Verification items for the finished model (mm, model axes). A direction names the side the tool comes from. Coordinates: 2 decimals unless noted, no trailing zeros. Loops run counter-clockwise (first coordinate to the right, second up) from the corner with the lowest first, then second, coordinate; pieces in that order, holes last. Notation, with made-up numbers: (63, 55.5) -> (105, 55.5) arc R19 ccw to (105, 82.5) -> close; hole circle Ø7 at (26, -5.75). An arc over 180 degrees is marked (long way). Answer as a JSON object with one key per item and string values. Group by question number.
Q1. Cross-section at C-C on y = 3053.5. Record the boundary of the cut face in (x, z).
Q2. Cross-section at B-B on x = 1900. Record the boundary of the cut face in (y, z).
Q3. Scan lines: L1, parallel to X at y = 3044.5, z = 2.9; L2, parallel to X at y = 3161, z = 3.2; L3, parallel to X at y = 2953, z = 4.55. Record each from-to range of solid material in increasing order.
Q4. Gauge pin test, flat ends, axial feed: pin 1 Ø3.5 at (x, y) = (1920.9, 2839.09) entering from +Z; pin 2 Ø2.5 at (x, z) = (1510, 3) entering from +Y; pin 3 Ø2.5 at (x, z) = (1641, 1.5) entering from -Y; pin 4 Ø1.5 at (x, z) = (1655, 3.5) entering from -Y. Record the tip position at first contact, or that the pin passes through.
Q5. Set-up check for faces 1 (the cylindrical face through (1470.405, 3112.471, 2.465)), 2 (the flat face through (1816.93, 3217.31, 2.46)): record each of +Z, -Z, +X, -X, +Y, -Y from which the full face is reachable in a straight line by a thin tool's end or side.
Q6. Cross-section at A-A on y = 3282. Give the number of separate pieces and of enclosed holes in the cut face, and give its area (3 significant figures).
```python
from build123d import *

# Parameters (mm, degrees)
MODEL_R         = 3
MODEL_R_2       = 2.999999999
EXTRUDE_1_DEPTH = 5


with BuildPart() as part:
    # Model → 凸台-拉伸1 (new body)
    with BuildSketch(Plane.XY):
        with BuildLine():
            Line((1801.04667122, 3384.62585133), (1652.053473941, 3384.62585133))
            ThreePointArc((1652.053473941, 3384.62585133), (1476.211681089, 3361.037418459), (1452.966845602, 3185.14987512))
            ThreePointArc((1452.966845602, 3185.14987512), (1470.408197338, 3111.400724011), (1452.966841198, 3037.651573943))
            ThreePointArc((1452.966841198, 3037.651573943), (1476.211684212, 2861.76403514), (1652.053473941, 2838.175605395))
            Line((1652.053473941, 2838.175605395), (1801.04667122, 2838.175605395))
            ThreePointArc((1801.04667122, 2838.175605395), (1976.888464071, 2861.764038266), (2000.13329956, 3037.651581604))
            ThreePointArc((2000.13329956, 3037.651581604), (1980.450087896, 3111.400728363), (2000.13329956, 3185.149875122))
            ThreePointArc((2000.13329956, 3185.149875122), (1976.888464071, 3361.037418459), (1801.04667122, 3384.62585133))
        make_face()
        with Locations((1463.462548046, 3185.149875121)):
            Circle(MODEL_R, mode=Mode.SUBTRACT)
        with Locations((1447.208426339, 3293.322313167)):
            Circle(MODEL_R, mode=Mode.SUBTRACT)
        with Locations((1525.324154834, 3383.712293191)):
            Circle(MODEL_R, mode=Mode.SUBTRACT)
        with Locations((1463.462548046, 3037.651582732)):
            Circle(MODEL_R, mode=Mode.SUBTRACT)
        with Locations((1447.208426339, 2929.479144686)):
            Circle(MODEL_R, mode=Mode.SUBTRACT)
        with Locations((1525.324154834, 2839.089164661)):
            Circle(MODEL_R, mode=Mode.SUBTRACT)
        with Locations((1991.691967871, 3185.149875121)):
            Circle(MODEL_R, mode=Mode.SUBTRACT)
        with Locations((2006.622075137, 3293.322313167)):
            Circle(MODEL_R, mode=Mode.SUBTRACT)
        with Locations((1920.899822368, 3383.712293191)):
            Circle(MODEL_R, mode=Mode.SUBTRACT)
        with Locations((1990.992539788, 3037.651582732)):
            Circle(MODEL_R, mode=Mode.SUBTRACT)
        with Locations((2007.92983358, 2929.479144686)):
            Circle(MODEL_R, mode=Mode.SUBTRACT)
        with Locations((1920.899822368, 2839.089164661)):
            Circle(MODEL_R, mode=Mode.SUBTRACT)
        with Locations((1723.111988601, 3372.896838033)):
            Circle(MODEL_R, mode=Mode.SUBTRACT)
        with Locations((1722.6694561, 2848.467983232)):
            Circle(MODEL_R, mode=Mode.SUBTRACT)
        with Locations((1579.55007258, 3257.900728363)):
            Circle(MODEL_R, mode=Mode.SUBTRACT)
        with Locations((1579.550072582, 2964.900728364)):
            Circle(MODEL_R_2, mode=Mode.SUBTRACT)
        with Locations((1872.548395989, 2963.902434755)):
            Circle(MODEL_R, mode=Mode.SUBTRACT)
        with Locations((1872.548395989, 3258.899021971)):
            Circle(MODEL_R, mode=Mode.SUBTRACT)
        with BuildLine():
            Line((1523.580291982, 3370.78732482), (1579.55007258, 3273.844821135))
            Line((1579.55007258, 3273.844821135), (1635.519853179, 3370.78732482))
            ThreePointArc((1635.519853179, 3370.78732482), (1579.55007258, 3383.900728363), (1523.580291982, 3370.78732482))
        make_face(mode=Mode.SUBTRACT)
        with BuildLine():
            Line((1509.772302601, 3362.815278434), (1565.742083199, 3265.872774749))
            Line((1565.742083199, 3265.872774749), (1453.802522002, 3265.872774749))
            ThreePointArc((1453.802522002, 3265.872774749), (1470.430871704, 3320.900728363), (1509.772302601, 3362.815278434))
        make_face(mode=Mode.SUBTRACT)
        with BuildLine():
            Line((1579.55007258, 3241.956635591), (1635.519853179, 3145.014131905))
            ThreePointArc((1635.519853179, 3145.014131905), (1579.55007258, 3131.900728363), (1523.580291982, 3145.014131905))
            Line((1523.580291982, 3145.014131905), (1579.55007258, 3241.956635591))
        make_face(mode=Mode.SUBTRACT)
        with BuildLine():
            Line((1593.358061961, 3249.928681977), (1649.32784256, 3152.986178291))
            ThreePointArc((1649.32784256, 3152.986178291), (1688.669273457, 3194.900728363), (1705.297623159, 3249.928681977))
            Line((1705.297623159, 3249.928681977), (1593.358061961, 3249.928681977))
        make_face(mode=Mode.SUBTRACT)
        with BuildLine():
            Line((1453.802522002, 3249.928681977), (1565.742083199, 3249.928681977))
            Line((1565.742083199, 3249.928681977), (1509.772302601, 3152.986178291))
            ThreePointArc((1509.772302601, 3152.986178291), (1470.430871704, 3194.900728363), (1453.802522002, 3249.928681977))
        make_face(mode=Mode.SUBTRACT)
        with BuildLine():
            Line((1649.32784256, 3362.815278434), (1593.358061961, 3265.872774749))
            Line((1593.358061961, 3265.872774749), (1705.297623159, 3265.872774749))
            ThreePointArc((1705.297623159, 3265.872774749), (1688.669273457, 3320.900728363), (1649.32784256, 3362.815278434))
        make_face(mode=Mode.SUBTRACT)
        with BuildLine():
            Line((1509.772302601, 2859.986179418), (1565.742083199, 2956.928683103))
            Line((1565.742083199, 2956.928683103), (1453.802522002, 2956.928683103))
            ThreePointArc((1453.802522002, 2956.928683103), (1470.430871328, 2901.900729155), (1509.772302601, 2859.986179418))
        make_face(mode=Mode.SUBTRACT)
        with BuildLine():
            Line((1579.55007258, 2980.844822261), (1635.519853179, 3077.787325947))
            ThreePointArc((1635.519853179, 3077.787325947), (1579.55007258, 3090.900729372), (1523.580291982, 3077.787325947))
            Line((1523.580291982, 3077.787325947), (1579.55007258, 2980.844822261))
        make_face(mode=Mode.SUBTRACT)
        with BuildLine():
            Line((1523.580291982, 2852.014133032), (1579.55007258, 2948.956636717))
            Line((1579.55007258, 2948.956636717), (1635.519853179, 2852.014133032))
            ThreePointArc((1635.519853179, 2852.014133032), (1579.55007258, 2838.900729372), (1523.580291982, 2852.014133032))
        make_face(mode=Mode.SUBTRACT)
        with BuildLine():
            Line((1593.358061961, 2972.872775875), (1649.32784256, 3069.815279561))
            ThreePointArc((1649.32784256, 3069.815279561), (1688.669273082, 3027.900729155), (1705.297623159, 2972.872775875))
            Line((1705.297623159, 2972.872775875), (1593.358061961, 2972.872775875))
        make_face(mode=Mode.SUBTRACT)
        with BuildLine():
            Line((1453.802522002, 2972.872775875), (1565.742083199, 2972.872775875))
            Line((1565.742083199, 2972.872775875), (1509.772302601, 3069.815279561))
            ThreePointArc((1509.772302601, 3069.815279561), (1470.430871329, 3027.900729588), (1453.802522002, 2972.872775875))
        make_face(mode=Mode.SUBTRACT)
        with BuildLine():
            Line((1649.32784256, 2859.986179418), (1593.358061961, 2956.928683103))
            Line((1593.358061961, 2956.928683103), (1705.297623159, 2956.928683103))
            ThreePointArc((1705.297623159, 2956.928683103), (1688.669273083, 2901.900729588), (1649.32784256, 2859.986179418))
        make_face(mode=Mode.SUBTRACT)
        with BuildLine():
            Line((1977.224599856, 2893.767619263), (1880.473351412, 2950.06736425))
            Line((1880.473351412, 2950.06736425), (1880.091966249, 2838.128452757))
            ThreePointArc((1880.091966249, 2838.128452757), (1935.176254316, 2854.569222229), (1977.224599856, 2893.767619263))
        make_face(mode=Mode.SUBTRACT)
        with BuildLine():
            Line((1856.604395758, 2963.956757288), (1759.853147314, 3020.256502275))
            ThreePointArc((1759.853147314, 3020.256502275), (1746.5491273, 2964.331724723), (1759.47176215, 2908.317590781))
            Line((1759.47176215, 2908.317590781), (1856.604395758, 2963.956757288))
        make_face(mode=Mode.SUBTRACT)
        with BuildLine():
            Line((1985.243644665, 2907.548367236), (1888.492396221, 2963.848112223))
            Line((1888.492396221, 2963.848112223), (1985.625029828, 3019.487278729))
            ThreePointArc((1985.625029828, 3019.487278729), (1998.547664678, 2963.473144788), (1985.243644665, 2907.548367236))
        make_face(mode=Mode.SUBTRACT)
        with BuildLine():
            Line((1864.623440566, 2977.73750526), (1767.872192123, 3034.037250247))
            ThreePointArc((1767.872192123, 3034.037250247), (1809.920537662, 3073.235647282), (1865.00482573, 3089.676416754))
            Line((1865.00482573, 3089.676416754), (1864.623440566, 2977.73750526))
        make_face(mode=Mode.SUBTRACT)
        with BuildLine():
            Line((1864.147966017, 2838.182775289), (1864.52935118, 2950.121686783))
            Line((1864.52935118, 2950.121686783), (1767.396717573, 2894.482520276))
            ThreePointArc((1767.396717573, 2894.482520276), (1809.176985627, 2854.998512196), (1864.147966017, 2838.182775289))
        make_face(mode=Mode.SUBTRACT)
        with BuildLine():
            Line((1977.700074405, 3033.322349234), (1880.567440798, 2977.683182728))
            Line((1880.567440798, 2977.683182728), (1880.948825962, 3089.622094221))
            ThreePointArc((1880.948825962, 3089.622094221), (1935.919806351, 3072.806357314), (1977.700074405, 3033.322349234))
        make_face(mode=Mode.SUBTRACT)
        with BuildLine():
            Line((1977.224599856, 3329.033837463), (1880.473351412, 3272.734092476))
            Line((1880.473351412, 3272.734092476), (1880.091966249, 3384.673003969))
            ThreePointArc((1880.091966249, 3384.673003969), (1935.176254316, 3368.232234498), (1977.224599856, 3329.033837463))
        make_face(mode=Mode.SUBTRACT)
        with BuildLine():
            Line((1856.604395758, 3258.844699439), (1759.853147314, 3202.544954452))
            ThreePointArc((1759.853147314, 3202.544954452), (1746.5491273, 3258.469732003), (1759.47176215, 3314.483865945))
            Line((1759.47176215, 3314.483865945), (1856.604395758, 3258.844699439))
        make_face(mode=Mode.SUBTRACT)
        with BuildLine():
            Line((1985.243644665, 3315.25308949), (1888.492396221, 3258.953344503))
            Line((1888.492396221, 3258.953344503), (1985.625029828, 3203.314177997))
            ThreePointArc((1985.625029828, 3203.314177997), (1998.547664678, 3259.328311939), (1985.243644665, 3315.25308949))
        make_face(mode=Mode.SUBTRACT)
        with BuildLine():
            Line((1864.623440566, 3245.063951466), (1767.872192123, 3188.764206479))
            ThreePointArc((1767.872192123, 3188.764206479), (1809.920537662, 3149.565809444), (1865.00482573, 3133.125039973))
            Line((1865.00482573, 3133.125039973), (1864.623440566, 3245.063951466))
        make_face(mode=Mode.SUBTRACT)
        with BuildLine():
            Line((1864.147966017, 3384.618681437), (1864.52935118, 3272.679769944))
            Line((1864.52935118, 3272.679769944), (1767.396717573, 3328.31893645))
            ThreePointArc((1767.396717573, 3328.31893645), (1809.176985627, 3367.80294453), (1864.147966017, 3384.618681437))
        make_face(mode=Mode.SUBTRACT)
        with BuildLine():
            Line((1977.700074405, 3189.479107492), (1880.567440798, 3245.118273999))
            Line((1880.567440798, 3245.118273999), (1880.948825962, 3133.179362505))
            ThreePointArc((1880.948825962, 3133.179362505), (1935.919806351, 3149.995099412), (1977.700074405, 3189.479107492))
        make_face(mode=Mode.SUBTRACT)
    extrude(amount=EXTRUDE_1_DEPTH)


solid = part.part
```
Computed values:
{
 "1": {"outline": "(1459.89, 0) -> (1489.96, 0) -> (1489.96, 5) -> (1459.89, 5) -> close; (1519.19, 0) -> (1537.6, 0) -> (1537.6, 5) -> (1519.19, 5) -> close; (1621.5, 0) -> (1639.91, 0) -> (1639.91, 5) -> (1621.5, 5) -> close; (1669.14, 0) -> (1783.96, 0) -> (1783.96, 5) -> (1669.14, 5) -> close; (1864.88, 0) -> (1880.83, 0) -> (1880.83, 5) -> (1864.88, 5) -> close; (1961.14, 0) -> (1992.25, 0) -> (1992.25, 5) -> (1961.14, 5) -> close"},
 "2": {"outline": "(2821.32, 0) -> (2840.93, 0) -> (2840.93, 5) -> (2821.32, 5) -> close; (2938.7, 0) -> (2957.15, 0) -> (2957.15, 5) -> (2938.7, 5) -> close; (2970.44, 0) -> (2988.81, 0) -> (2988.81, 5) -> (2970.44, 5) -> close; (3086.88, 0) -> (3135.93, 0) -> (3135.93, 5) -> (3086.88, 5) -> close; (3233.99, 0) -> (3252.36, 0) -> (3252.36, 5) -> (3233.99, 5) -> close; (3265.65, 0) -> (3284.1, 0) -> (3284.1, 5) -> (3265.65, 5) -> close; (3381.87, 0) -> (3401.48, 0) -> (3401.48, 5) -> (3381.87, 5) -> close"},
 "3": {"L1": "x = 1456.2 to 1481.88, 1524.39 to 1542.8, 1616.3 to 1634.71, 1677.22 to 1775.7, 1864.85 to 1880.8, 1969.4 to 1996.43", "L2": "x = 1462.76 to 1499.01, 1514.4 to 1532.81, 1626.29 to 1644.7, 1660.09 to 1793.23, 1864.91 to 1880.85, 1951.87 to 1989.01", "L3": "x = 1434.04 to 1454.11, 1563.47 to 1595.63, 1704.99 to 1747.02, 1837.48 to 1907.13, 1998.08 to 2019.06"},
 "4": {"pin 1": "passes through", "pin 2": "stops at y = 3386.94", "pin 3": "stops at y = 2831.89", "pin 4": "stops at y = 2838.18"},
 "5": {"face 1": "+Z, -Z, -X", "face 2": "+Z, -Z"},
 "6": {"separate pieces": "8", "enclosed holes": "0", "area": "1,020 mm²"}
}
